from build123d import *

# Parameters (mm, degrees)
CYLINDER_R                     = 1.25
CYLINDER_DEPTH                 = 10
CYLINDER_ROLL_ANGLE            = 90
REVOLVE_ONTO_SKETCH_ROLL_ANGLE = 90


with BuildPart() as setscrew_drill:
    # Cylinder → Cylinder (new body)
    with BuildSketch(Plane.XY):
        Circle(CYLINDER_R)
    extrude(amount=CYLINDER_DEPTH)


with BuildPart() as setscrew_drill_1:
    # Cylinder roll: moved
    add(setscrew_drill.part.rotate(Axis((0, 0, 0), (1, 0, 0)), CYLINDER_ROLL_ANGLE))


with BuildPart() as setscrew_drill_2:
    # Cylinder placement: moved
    add(setscrew_drill_1.part.moved(Location((0, 0, 3))))


with BuildPart() as extruder_drive_gear:
    # Sketch as drawn → Revolve (revolve)
    with BuildSketch(Plane.XY):
        with BuildLine():
            Line((-6.25, 5), (-6.25, 0))
            Line((-6.25, 0), (-2.5, 0))
            Line((-2.5, 0), (-2.5, 11))
            Line((-2.5, 11), (-6.25, 11))
            Line((-6.25, 11), (-6.25, 9))
            ThreePointArc((-6.25, 5), (-5.25, 7), (-6.25, 9))
        make_face()
    revolve(axis=Axis((0, 0, 0), (0, 1, 0)))


with BuildPart() as extruder_drive_gear_1:
    # Revolve onto Sketch roll: moved
    add(extruder_drive_gear.part.rotate(Axis((0, 0, 0), (1, 0, 0)), REVOLVE_ONTO_SKETCH_ROLL_ANGLE))


with BuildPart() as extruder_drive_gear_2:
    # Revolve onto Sketch placement: moved
    add(extruder_drive_gear_1.part)

    # Cut: cut setscrew-drill
    add(setscrew_drill_2.part, mode=Mode.SUBTRACT)


solid = extruder_drive_gear_2.part
Read the model definition and answer for the solid it produces. Units are mm, in the model's axes. Round coordinates to 2 decimals unless told otherwise and drop trailing zeros. Write each loop counter-clockwise with the first axis right and the second up, starting at its lowest first coordinate (ties: lowest second). Pieces come first, ordered by that corner, then holes.
Q1. Straight lines are drawn through the part: line 1 (Z direction, x = 0, y = -4.5); line 2 (Z direction, x = -5, y = -2.25); line 3 (Y direction, x = -1.5, z = 1.75). For each, find the intervals that lie inside material, in ascending order.
Values:
line 1: z = 0 to 1.75, 4.25 to 11
line 2: z = 0 to 5.95, 8.05 to 11
line 3: y = -6.07 to -2, 2 to 6.07
Q2. Find section B-B on z = 7. Determine the outline of the cut face in (x, y), and give its area (3 significant figures).
Values:
outline: circle Ø10.5 at (0, 0); hole circle Ø5 at (0, 0)
area: 67.0 mm2
Q3. Find section A-A on y = 0. Determine the outline of the cut face in (x, z), and give its area (3 significant figures).
Values:
outline: (-6.25, 0) - (-2.5, 0) - (-2.5, 11) - (-6.25, 11) - (-6.25, 9) arc R2.5 cw to (-6.25, 5) - close; (2.5, 0) - (6.25, 0) - (6.25, 5) arc R2.5 cw to (6.25, 9) - (6.25, 11) - (2.5, 11) - close
area: 76.9 mm2
Q4. Find section D-D on z = 3. Determine the outline of the cut face in (x, y), and give its area (3 significant figures).
Values:
outline: (-1.25, -6.12) - (-1.25, -2.17) arc R2.5 cw (long way) to (1.25, -2.17) - (1.25, -6.12) arc R6.25 ccw (long way) to start
area: 93.5 mm2
Q5. Find section C-C on z = 9.25. Determine the outline of the cut face in (x, y), and give its area (3 significant figures).
Values:
outline: circle Ø12.5 at (0, 0); hole circle Ø5 at (0, 0)
area: 103 mm2
Q6. Flat-ended cylindrical pins translate along their axes: P1, Ø1.5, axis at y = 4, z = 2.5, coming from the -X side; P2, Ø4, axis at x = 0, y = 0, coming from the +Z side; P3, Ø2, axis at x = -3.5, z = 1.5, coming from the +Y side; P4, Ø6, axis at x = -3.5, z = 7.5, coming from the -Y side. Find the tip coordinate at first contact, or state that the pin passes through.
Values:
P1: stops at x = -5.34
P2: passes through
P3: stops at y = 5.73
P4: stops at y = -6.18
Q7. The mould has two halves that part along Z. Classify faces 1 (the face through (0, 3, 0)), 2 (the face through (-1.25, -4.18, 3.05)), 3 (the face through (-5.96, -1.88, 9.99)): released by +Z, released by -Z, zero draft, split by the parting line, or undercut.
Values:
face 1: released by -Z
face 2: undercut
face 3: zero draft
